```python
from build123d import *

# Parameters (mm, degrees)
BOSS_EXTRUDE2_DEPTH = 110
SKETCH2_R           = 5
CUT_EXTRUDE1_DEPTH  = 543.741338024
SKETCH3_W           = 10
SKETCH3_H           = 110
BOSS_EXTRUDE3_DEPTH = 25
SKETCH5_R           = 30
CUT_EXTRUDE2_DEPTH  = 543.741338024


with BuildPart() as part:
    # Sketch1 → Boss-Extrude2 (new body)
    with BuildSketch(Plane.XY):
        with BuildLine():
            Line((20, 29.6), (510, 29.6))
            ThreePointArc((510, 29.6), (517.071067812, 26.671067812), (520, 19.6))
            Line((520, 19.6), (520, 0))
            Line((520, 0), (530, 0))
            Line((530, 0), (530, 19.6))
            ThreePointArc((530, 19.6), (524.142135624, 33.742135624), (510, 39.6))
            Line((510, 39.6), (20, 39.6))
            ThreePointArc((20, 39.6), (5.857864376, 33.742135624), (0, 19.6))
            Line((0, 19.6), (0, 0))
            Line((0, 0), (10, 0))
            Line((10, 0), (10, 19.6))
            ThreePointArc((10, 19.6), (12.928932188, 26.671067812), (20, 29.6))
        make_face()
    extrude(amount=BOSS_EXTRUDE2_DEPTH)

    # Sketch2 → Cut-Extrude1 (cut, through all)
    with BuildSketch(Plane.ZY):
        with Locations((30, 10)):
            Circle(SKETCH2_R)
        with Locations(Location((80, 10, 0), (0, 0, 180))):
            Circle(SKETCH2_R)
    extrude(amount=-CUT_EXTRUDE1_DEPTH, mode=Mode.SUBTRACT)

    # Sketch3 → Boss-Extrude3 (add)
    with BuildSketch(Plane(origin=(0, 39.6, 0), x_dir=(1, 0, 0), z_dir=(0, 1, 0))):
        with Locations((225, -55)):
            Rectangle(SKETCH3_W, SKETCH3_H)
        with Locations((305, -55)):
            Rectangle(SKETCH3_W, SKETCH3_H)
    extrude(amount=BOSS_EXTRUDE3_DEPTH)

    # Sketch5 → Cut-Extrude2 (cut, through all)
    with BuildSketch(Plane(origin=(0, 39.6, 0), x_dir=(1, 0, 0), z_dir=(0, 1, 0))):
        with Locations(Location((264.500885843, -69, 0), (0, 0, 270))):
            Circle(SKETCH5_R)
    extrude(amount=-CUT_EXTRUDE2_DEPTH, mode=Mode.SUBTRACT)


solid = part.part
```
For this review, take the finished solid that the model builds, in its own axes (mm). A direction names the side the tool comes from. Give positions to 0.01 mm unless a question says otherwise; leave off trailing zeros. Write each loop counter-clockwise with the first axis right and the second up, starting at its lowest first coordinate (ties: lowest second). Pieces come first, ordered by that corner, then holes.
Item 1: Take a section at B-B (z = 30). Give the boundary of the cut face in (x, y), and give its area (3 significant figures).
Item 2: Take a section at C-C (y = 49). Give the boundary of the cut face in (x, z).
Item 3: The part is to be moulded in two halves that separate along X. For faces 1 (the face through (4.93, 11.915, 75.381)), 2 (the face through (0, 10, 54)), 3 (the face through (235.214, 34.67, 62.497)), say which applies: +X half, -X half, draft (parallel to the pull), parting line (faces both ways), or undercut.
Item 4: Take a section at A-A (z = 69). Give the boundary of the cut face in (x, y), and give its area (3 significant figures).
Item 5: Take a section at D-D (x = 497.5). Give the boundary of the cut face in (y, z), and give its area (3 significant figures).
Item 6: Wall thickness on probe 1 along X at (y, z) = (46, 36); probe 2 along X at (y, z) = (16.5, 96); probe 3 along Y at (x, z) = (469, 89.5): over which ranges is each line inside the solid? List them lowest first.
Item 7: Insertion check: P1, Ø16, axis at y = 10, z = 80, coming from the +X side; P2, Ø1, axis at x = 141.5, z = 86.5, coming from the +Y side; P3, Ø10, axis at y = 26.5, z = 12.5, coming from the -X side; P4, Ø1, axis at x = 190, z = 45.5, coming from the -Y side. Each pin has a flat end and moves straight along its axis. Give the tip position at first contact, or say it passes through.
Item 8: Machinability: for faces 4 (the face through (220, 52, 56)), 5 (the face through (520, 10, 54)), 6 (the face through (244, 32, 0)), 7 (the face through (230, 52, 56)), 8 (the face through (411, 39.6, 54)), which of the approach directions +Z, -Z, +X, -X, +Y, -Y give a long, thin tool a straight path to every point of the face, cutting with its end or side? Answer none if there is none.
Established:
1. outline: (0, 0) - (10, 0) - (10, 5) - (0, 5) - close; (0, 15) - (10, 15) - (10, 19.6) arc R10 cw to (20, 29.6) - (510, 29.6) arc R10 cw to (520, 19.6) - (520, 15) - (530, 15) - (530, 19.6) arc R20 ccw to (510, 39.6) - (310, 39.6) - (310, 64.6) - (300, 64.6) - (300, 39.6) - (230, 39.6) - (230, 64.6) - (220, 64.6) - (220, 39.6) - (20, 39.6) arc R20 ccw to (0, 19.6) - close; (520, 0) - (530, 0) - (530, 5) - (520, 5) - close
1. area: 6,060 mm2
2. outline: (220, 0) - (230, 0) - (230, 110) - (220, 110) - close; (300, 0) - (310, 0) - (310, 110) - (300, 110) - close
3. face 1: draft
3. face 2: -X half
3. face 3: undercut
4. outline: (0, 0) - (10, 0) - (10, 19.6) arc R10 cw to (20, 29.6) - (234.5, 29.6) - (234.5, 39.6) - (230, 39.6) - (230, 64.6) - (220, 64.6) - (220, 39.6) - (20, 39.6) arc R20 ccw to (0, 19.6) - close; (294.5, 29.6) - (510, 29.6) arc R10 cw to (520, 19.6) - (520, 0) - (530, 0) - (530, 19.6) arc R20 ccw to (510, 39.6) - (310, 39.6) - (310, 64.6) - (300, 64.6) - (300, 39.6) - (294.5, 39.6) - close
4. area: 5,660 mm2
5. outline: (29.6, 0) - (39.6, 0) - (39.6, 110) - (29.6, 110) - close
5. area: 1,100 mm2
6. probe 1: x = 220 to 230, 300 to 310
6. probe 2: x = 0 to 10, 520 to 530
6. probe 3: y = 29.6 to 39.6
7. P1: stops at x = 530
7. P2: stops at y = 39.6
7. P3: stops at x = 0.09
7. P4: stops at y = 29.6
8. face 4: +Z, -Z, -X, +Y
8. face 5: +Z, -Z, -Y
8. face 6: -Z, +X, -X, +Y, -Y
8. face 7: +Z, -Z, +Y
8. face 8: +Z, -Z, +X, +Y
